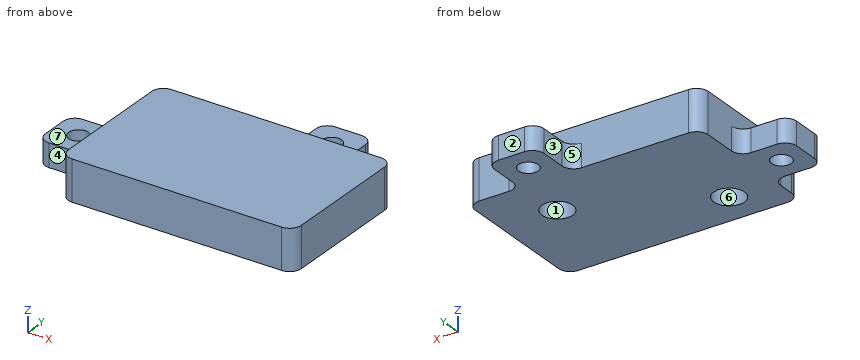
Autodesk Fusion 360 part; units mm, degrees
sketch "Sketch1" plane through (0, 0, 0) normal (0, 0, 1) x (1, 0, 0)
  line L0 (0, 0) -> (0, 10.5)
  line L1 (0, 0) -> (22.3571, 10.5)
  circle A0 centre (0, 0) radius 2 construction
  circle A1 centre (22.3571, 10.5) radius 2 construction
  line L2 (-8, -6) -> (32, -6)
  line L3 (32, -6) -> (32, 19)
  line L4 (32, 19) -> (-8, 19)
  line L5 (-8, 19) -> (-8, -6)
  dimension "d1" = 10.5
  dimension "d2" = 24.7
  dimension "d3" = 4
  dimension "d4" = 4
  dimension "d5" = 25
  dimension "d6" = 40
  dimension "d7" = 8
  dimension "d8" = 6
extrude "Extrude1" add sketch "Sketch1" along normal blind 3 makes body 1
sketch "Sketch2" plane through (0, 0, 0) normal (0, 0, 1) x (1, 0, 0)
  circle A0 centre (0, 0) radius 2.65
  circle A1 centre (22.3571, 10.5) radius 2.65
  point P0 (22.3571, 10.5)
  dimension "d11" = 5.3
  dimension "d12" = 5.3
extrude "Extrude2" cut sketch "Sketch2" along normal blind 2 bodies 1
hole "Hole1" at (-22.3571, -10.5, 2) direction (0, 0, 1) diameter 3.4 depth 4 tip angle 118 bodies 1
sketch "Sketch4" plane through (0, 0, 0) normal (0, 0, -1) x (1, 0, 0)
  circle A0 centre (0, 0) radius 2.65
  line L0 (-8, 6) -> (-8, -19)
  line L1 (-8, -19) -> (32, -19)
  line L2 (32, -19) -> (32, 6)
  line L3 (32, 6) -> (-8, 6)
  line L4 (-12.2925, -4.85) -> (18.65, -23.25) construction
  line L5 (-8, -0.65) -> (-16.5, -0.65)
  line L6 (-16.5, -0.65) -> (-16.5, -9.15)
  line L7 (-16.5, -9.15) -> (-8, -9.15)
  line L8 (-8, -9.15) -> (-8, -0.65)
  line L9 (-16.5, -4.9) -> (-8, -4.9) construction
  line L10 (14.4, -19) -> (22.9, -19) construction
  line L11 (22.9, -19) -> (22.9, -27.5)
  line L12 (22.9, -27.5) -> (14.4, -27.5)
  line L13 (14.4, -27.5) -> (14.4, -19)
  line L14 (18.65, -19) -> (18.65, -27.5) construction
  line L15 (22.9, -23.25) -> (14.4, -23.25) construction
  line L16 (-12.25, -9.15) -> (-12.25, -0.65) construction
  dimension "d26" = 36
  dimension "d27" = 18.4
  dimension "d28" = 8.5
  dimension "d29" = 8.5
  dimension "d30" = 9.85
  dimension "d31" = 8.5
  dimension "d32" = 8.5
  dimension "d42" = 9.1
extrude "Extrude3" add sketch "Sketch4" along normal blind 4 separate body contours L0 L5 L6 L7 L8 | L1 L11 L12 L13 makes body 2 at (-10.8333, 3.4833, 0) makes body 3 at (17.2333, 24.6667, 0)
extrude "Extrude4" add 1 faces at (4.2643, 10.916, 0) along direction (0, 0, -1) up to surface (4 mm away) on bodies 1 bodies 1 2 3
hole "Hole3" at (18.65, 23.25, 0) at (-12.2925, 4.85, 0) direction (0, 0, -1) diameter 3.4 depth 4 tip angle 118 bodies 1
extrude "Extrude7" add 1 faces at (-0.1169, 0.6581, 2) along direction (0, 0, -1) blind 1 on bodies 1 bodies 1
fillet "Fillet1" radius 2 12 edges at (-8, 0.65, -2) (-16.5, 0.65, -2) (-8, 9.15, -2) (-16.5, 9.15, -2) (14.4, 19, -2) (22.9, 19, -2) (22.9, 27.5, -2) (14.4, 27.5, -2) (-8, -6, -0.5) (32, -6, -0.5) (32, 19, -0.5) (-8, 19, -0.5) on bodies 1
The model under review builds one solid part; all positions refer to its coordinate system, in mm. Face numbers are marked on the shaded views. A direction names the side the tool comes from. Give positions to 0.01 mm unless a question says otherwise; leave off trailing zeros. Write each loop counter-clockwise with the first axis right and the second up, starting at its lowest first coordinate (ties: lowest second). Pieces come first, ordered by that corner, then holes. Notation, with made-up numbers: M 24.5,33 L 64.5,33 A10 ccw 64.5,42 Z; hole C -17.75,-25 d2. An arc over 180 degrees is marked long. One line per question, with ' | ' between items. Start each with the question number.
Item 1: We need section D-D on z = -2.5. Write out the cut boundary in (x, y), plus the area to 3 significant figures.
Item 2: Wall thickness on line 1 (X direction, y = 23.25, z = -2.85); line 2 (Y direction, x = 18.65, z = -1.45); line 3 (X direction, y = 4.85, z = -3): over which ranges is each line inside the solid? List them lowest first. Write a range as from..to.
Item 3: We need section C-C on x = 0. Write out the cut boundary in (y, z), plus the area to 4 significant figures.
Item 4: We need section B-B on z = 1.5. Write out the cut boundary in (x, y).
Item 5: For the marked faces 1, 2, 3 and 4, list the 3-axis set-ups (+Z, -Z, +X, -X, +Y, -Y) from which the entire face can be reached by the end or side of a thin tool; tool diameter is ignored.
Item 6: Draft analysis for pull direction X (two halves, no side actions). For the marked faces 5, 6 and 7, state which applies: released by +X, released by -X, zero draft, split by the parting line, or undercut.
Item 7: We need section A-A on y = 4.85. Write out the cut boundary in (x, z).
Item 8: For pin 1 (1.2 mm diameter, centred on x = -13, z = -3, fed in from -Y); pin 2 (4 mm diameter, centred on x = 22, y = 10, fed in from -Z); pin 3 (1.5 mm diameter, centred on y = -2, z = 0.5, fed in from -X), all flat-tipped, find the tip position at first contact; note any pin that passes through.
Results found:
1) outline: M -16.5,2.65 A2 ccw -14.5,0.65 L -10,0.65 A2 cw -8,-1.35 L -8,-4 A2 ccw -6,-6 L 30,-6 A2 ccw 32,-4 L 32,17 A2 ccw 30,19 L 24.9,19 A2 cw 22.9,21 L 22.9,25.5 A2 ccw 20.9,27.5 L 16.4,27.5 A2 ccw 14.4,25.5 L 14.4,21 A2 cw 12.4,19 L -6,19 A2 ccw -8,17 L -8,11.15 A2 cw -10,9.15 L -14.5,9.15 A2 ccw -16.5,7.15 Z; hole C -12.29,4.85 d3.4; hole C 0,0 d5.3; hole C 18.65,23.25 d3.4; hole C 22.36,10.5 d5.3 | area: 1,080 mm2
2) line 1: x = 14.4..16.95, 20.35..22.9 | line 2: y = -6..21.55, 24.95..27.5 | line 3: x = -16.5..-13.99, -10.59..32
3) outline: M -6,-4 L -2.65,-4 L -2.65,1 L 2.65,1 L 2.65,-4 L 19,-4 L 19,3 L -6,3 Z | area: 148.5 mm2
4) outline: M -8,-4 A2 ccw -6,-6 L 30,-6 A2 ccw 32,-4 L 32,17 A2 ccw 30,19 L -6,19 A2 ccw -8,17 Z; hole C 22.36,10.5 d5.3
5) face 1: -Z | face 2: +Z, -Z, +X, -X, +Y | face 3: +Z, -Z, -X, +Y | face 4: +Z, -Z, -X, -Y
6) face 5: released by -X | face 6: undercut | face 7: zero draft
7) outline: M -16.5,-4 L -13.99,-4 L -13.99,0 L -16.5,0 Z; M -10.59,-4 L 32,-4 L 32,3 L -8,3 L -8,0 L -10.59,0 Z
8) pin 1: stops at y = 0.65 | pin 2: stops at z = 2 | pin 3: stops at x = -8
